The listing builds one solid part. Answer for the finished solid, in the listing's coordinates (mm). A direction names the side the tool comes from. Coordinates: 2 decimals unless noted, no trailing zeros. Loops run counter-clockwise (first coordinate to the right, second up) from the corner with the lowest first, then second, coordinate; pieces in that order, holes last. Notation, with made-up numbers: (-17.75, 17.5) - (-10.75, 17.5) arc R23 cw to (-10.75, 36.5) - close; hole circle Ø5 at (82, -28.75). An arc over 180 degrees is marked (long way). Use one line per item in the form item = value. Start each with the question number.
```python
from build123d import *

# Parameters (mm, degrees)
SKETCH1_W               = 16.4
SKETCH1_H               = 26.4
SKETCH1_W_2             = 12.4
SKETCH1_H_2             = 22.4
BOSS_EXTRUDE1_DEPTH     = 20
CUT_EXTRUDE1_DEPTH      = 10
BOSS_EXTRUDE2_DEPTH     = 3
CHAMFER3_SIZE           = 0.4
SKETCH5_W               = 2
SKETCH5_H               = 14.997550085
BOSS_EXTRUDE3_DEPTH     = 10
LPATTERN1_COUNT         = 2
LPATTERN1_PITCH         = 17
CHAMFER1_SIZE           = 0.4
CHAMFER5_SIZE           = 0.4
CHAMFER6_SIZE           = 0.4
CUT_EXTRUDE2_DEPTH      = 47.301249176
CUT_EXTRUDE2_DEPTH_BACK = 47.301249176
SKETCH6_W               = 6.042108652
SKETCH6_H               = 2


with BuildPart() as part:
    # Sketch1 → Boss-Extrude1 (new body)
    with BuildSketch(Plane(origin=(0, 0, 0), x_dir=(1, 0, 0), z_dir=(0, 1, 0))):
        with Locations((6.2, 11.2)):
            Rectangle(SKETCH1_W, SKETCH1_H)
        with Locations((6.2, 11.2)):
            Rectangle(SKETCH1_W_2, SKETCH1_H_2, mode=Mode.SUBTRACT)
    extrude(amount=BOSS_EXTRUDE1_DEPTH)

    # Sketch2 → Cut-Extrude1 (cut)
    with BuildSketch(Plane(origin=(0, 0, -24.4), x_dir=(-1, 0, 0), z_dir=(0, 0, -1))):
        Polygon((-12.4, 20), (-12.4, 17.712061235), (-10.544532553, 15.856593788), (-9.258136531, 15.293507674), (-9.258136531, 13.764128217), (-8.084426715, 12.5904184), (-6.2, 11.765560038), (-4.315573285, 12.5904184), (-3.141863469, 13.764128217), (-3.141863469, 15.293507674), (-1.855467447, 15.856593788), (0, 17.712061235), (0, 20), align=None)
    extrude(amount=-CUT_EXTRUDE1_DEPTH, mode=Mode.SUBTRACT)



with BuildPart() as body_2:
    # Sketch4 → Boss-Extrude2 (new body)
    with BuildSketch(Plane(origin=(0, 30, 0), x_dir=(1, 0, 0), z_dir=(0, 1, 0))):
        Polygon((12.4, 12.2), (14.4, 12.2), (14.4, 39.19752129), (12.472658245, 39.19752129), (7.96501827, 39.19752129), (5.96501827, 39.19752129), (5.96501827, 33.473580557), (7.96501827, 33.473580557), (7.96501827, 37.19752129), (9.06501827, 37.19752129), (9.06501827, 36.19752129), (10.06501827, 36.19752129), (10.06501827, 37.19752129), (12.06501827, 37.19752129), (12.06501827, 27.08752129), (10.06501827, 27.08752129), (10.06501827, 28.08752129), (9.06501827, 28.08752129), (9.06501827, 24.08752129), (12.4, 24.08752129), align=None)
    boss_extrude2 = extrude(amount=-BOSS_EXTRUDE2_DEPTH)

    # Chamfer3
    chamfer3_edges = [body_2.edges().sort_by_distance(p)[0] for p in [
        (6.96501827, 27, -33.473580557),
        (7.96501827, 27, -35.335550923),
        (8.51501827, 27, -37.19752129),
        (9.06501827, 27, -36.69752129),
        (9.56501827, 27, -36.19752129),
        (10.06501827, 27, -36.69752129),
        (11.06501827, 27, -37.19752129),
        (9.56501827, 27, -28.08752129),
        (10.06501827, 27, -27.58752129),
        (11.06501827, 27, -27.08752129),
        (12.06501827, 27, -32.14252129),
    ]]
    chamfer(chamfer3_edges, length=CHAMFER3_SIZE)


with BuildPart() as part_1:
    add(part.part)

    add(body_2.part)  # Boss-Extrude3 merges body 2
    # Sketch5 → Boss-Extrude3 (add)
    with BuildSketch(Plane(origin=(0, 30, 0), x_dir=(1, 0, 0), z_dir=(0, 1, 0))):
        with Locations((13.4, 16.588746248)):
            Rectangle(SKETCH5_W, SKETCH5_H)
    extrude(amount=-BOSS_EXTRUDE3_DEPTH)

    # LPattern1: Boss-Extrude2 ×2
    with Locations(*[(0, -i * LPATTERN1_PITCH, 0) for i in range(1, LPATTERN1_COUNT)]):
        add(boss_extrude2)

    # Chamfer1
    chamfer1_edges = [part_1.edges().sort_by_distance(p)[0] for p in [
        (9.56501827, 30, -28.08752129),
        (10.06501827, 30, -27.58752129),
        (7.96501827, 30, -35.335550923),
        (8.51501827, 30, -37.19752129),
        (9.06501827, 30, -36.69752129),
        (9.56501827, 30, -36.19752129),
        (10.06501827, 30, -36.69752129),
        (11.06501827, 30, -27.08752129),
        (11.06501827, 30, -37.19752129),
        (12.06501827, 30, -32.14252129),
    ]]
    chamfer(chamfer1_edges, length=CHAMFER1_SIZE)

    # Chamfer5
    chamfer5_edges = [part_1.edges().sort_by_distance(p)[0] for p in [
        (6.96501827, 10, -33.473580557),
        (7.96501827, 10, -35.335550923),
        (8.51501827, 10, -37.19752129),
        (9.06501827, 10, -36.69752129),
        (9.56501827, 10, -36.19752129),
        (10.06501827, 10, -36.69752129),
        (11.06501827, 10, -37.19752129),
        (12.06501827, 10, -32.14252129),
        (11.06501827, 10, -27.08752129),
    ]]
    chamfer(chamfer5_edges, length=CHAMFER5_SIZE)

    # Chamfer6
    chamfer6_edges = [part_1.edges().sort_by_distance(p)[0] for p in [
        (9.06501827, 28.5, -28.08752129),
        (10.06501827, 28.5, -28.08752129),
        (10.06501827, 28.5, -36.19752129),
        (9.06501827, 28.5, -36.19752129),
        (10.06501827, 11.7, -36.19752129),
        (9.06501827, 11.7, -36.19752129),
        (9.06501827, 11.5, -28.08752129),
    ]]
    chamfer(chamfer6_edges, length=CHAMFER6_SIZE)

    # Sketch6 → Cut-Extrude2 (cut, two sides: drawn at the far end of the back side and taken through both)
    with BuildSketch(Plane(origin=(0, 20, 0), x_dir=(1, 0, 0), z_dir=(0, 1, 0)).offset(-CUT_EXTRUDE2_DEPTH_BACK)):
        with Locations((6.2, -1)):
            Rectangle(SKETCH6_W, SKETCH6_H)
    extrude(amount=CUT_EXTRUDE2_DEPTH + CUT_EXTRUDE2_DEPTH_BACK, mode=Mode.SUBTRACT)


solid = part_1.part
```
(1) A cutting plane is placed at A-A (z = -32). Determine the outline of the cut face in (x, y), then the cut area to 3 significant figures.
(2) Find the intervals of material crossed by probe 1 along Z at (x, y) = (10.5, 3.5); probe 2 along X at (y, z) = (18, -18); probe 3 along Y at (x, z) = (6.75, -36), in increasing order. Write a range as from..to.
(3) Each of these flat-tipped pins is pushed along its axis until it touches: pin 1 Ø1.6 at (x, y) = (13, 24) entering from -Z; pin 2 Ø1.5 at (y, z) = (22, -5.5) entering from +X; pin 3 Ø4 at (x, z) = (11, -2.5) entering from +Y; pin 4 Ø8 at (x, y) = (6.5, 26) entering from +Z. Where does it stop, or does it pass through?
(4) For faces 1 (the face through (13, 13, -32)), 2 (the face through (3.179, 10, 1)), 3 (the face through (11, 29, -37.198)), 4 (the face through (11, 29, -24.088)), 5 (the face through (14.4, 15, -14)), determine the directions among +Z, -Z, +X, -X, +Y, -Y from which every point of the face is accessible in a straight line to the end or side of a thin tool.
(5) A cutting plane is placed at B-B (y = 6). Determine the outline of the cut face in (x, z), then the cut area to 3 significant figures.
(6) A cutting plane is placed at D-D (z = -4). Determine the outline of the cut face in (x, y), then the cut area to 3 significant figures.
(7) Determine the mould class of faces 6 (the face through (13, 10, -34)), 7 (the face through (13, 27, -33)), 8 (the face through (11, 12, -37.198)) for opening direction Y: +Y half, -Y half, draft (parallel to the pull), parting line (faces both ways), or undercut.
(8) A cutting plane is placed at C-C (x = 6.75). Determine the outline of the cut face in (y, z), then the cut area to 3 significant figures.
Evaluation:
q1.outline = (12.07, 10.4) - (12.47, 10) - (14.4, 10) - (14.4, 13) - (12.07, 13) - close; (12.07, 27.4) - (12.47, 27) - (14.4, 27) - (14.4, 30) - (12.47, 30) - (12.07, 29.6) - close
q1.area = 13.8 mm^2
q2.probe_1 = -24.4..-22.4, 0..2
q2.probe_2 = -2..0, 12.4..14.4
q2.probe_3 = 10..13, 27..30
q3.pin_1 = -24.09
q3.pin_2 = through
q3.pin_3 = 20
q3.pin_4 = -24.09
q4.face_1 = -Z, +X, -X
q4.face_2 = +Z, +Y, -Y
q4.face_3 = +Y, -Y
q4.face_4 = +Z, -X, +Y
q4.face_5 = +Z, -Z, +X, +Y, -Y
q5.outline = (-2, -24.4) - (14.4, -24.4) - (14.4, 2) - (9.22, 2) - (9.22, 0) - (12.4, 0) - (12.4, -22.4) - (0, -22.4) - (0, 0) - (3.18, 0) - (3.18, 2) - (-2, 2) - close
q5.area = 143 mm^2
q6.outline = (-2, 0) - (0, 0) - (0, 20) - (-2, 20) - close; (12.4, 0) - (14.4, 0) - (14.4, 20) - (12.4, 20) - close
q6.area = 80.0 mm^2
q7.face_6 = -Y half
q7.face_7 = undercut
q7.face_8 = draft
q8.outline = (0, -24.4) - (12.01, -24.4) - (12.01, -22.4) - (0, -22.4) - close; (10, -39.2) - (13, -39.2) - (13, -33.47) - (10.4, -33.47) - (10, -33.87) - close; (27, -39.2) - (30, -39.2) - (30, -33.47) - (27.4, -33.47) - (27, -33.87) - close
q8.area = 58.2 mm^2
